Design review of the part built by this model. Coordinates are the model's own, in mm. Face numbers are marked on the shaded views. A direction names the side the tool comes from. Give positions to 0.01 mm unless a question says otherwise; leave off trailing zeros. Loops run counter-clockwise (first coordinate to the right, second up) from the corner with the lowest first, then second, coordinate; pieces in that order, holes last. Notation, with made-up numbers: (2.5, -38) - (53.5, -38) arc R6 cw to (53.5, -29) - close; hole circle Ø9 at (-9.5, -21.5). An arc over 180 degrees is marked (long way). Write each question's results on one line, items separated by ' | '.
```python
from build123d import *

# Parameters (mm, degrees)
SKETCH1_R               = 37.846
SKETCH1_R_2             = 14.224
BOSS_EXTRUDE1_DEPTH     = 6.35
CUT_EXTRUDE1_DEPTH      = 1
CUT_EXTRUDE1_DEPTH_BACK = 7.35
CUT_EXTRUDE2_DEPTH      = 1
CUT_EXTRUDE2_DEPTH_BACK = 7.35


with BuildPart() as part:
    # Sketch1 → Boss-Extrude1 (new body)
    with BuildSketch(Plane(origin=(0, 0, 0), x_dir=(1, 0, 0), z_dir=(0, 1, 0))):
        Circle(SKETCH1_R)
        Circle(SKETCH1_R_2, mode=Mode.SUBTRACT)
    extrude(amount=BOSS_EXTRUDE1_DEPTH)

    # Sketch2 → Cut-Extrude1 (cut, two sides)
    with BuildSketch(Plane(origin=(0, 6.35, 0), x_dir=(1, 0, 0), z_dir=(0, 1, 0))) as cut_extrude1_sk:
        Polygon((-18.723278008, -3.767243493), (-19.849678423, -4.7625), (-22.882156733, -4.7625), (-24.01035364, -3.767243493), (-24.01035364, -2.234835911), (-22.294703885, -2.234835911), (-22.294703885, -3.00373444), (-20.480247077, -3.00373444), (-20.480247077, -0.882077518), (-22.93605149, -0.882077518), (-24.058858921, 0.113178989), (-24.058858921, 3.761854017), (-22.93605149, 4.7625), (-19.862253866, 4.7625), (-18.723278008, 3.756464542), align=None)
        Polygon((-24.955308374, -3.767243493), (-26.083505281, -4.7625), (-29.139337986, -4.7625), (-30.267534892, -3.767243493), (-30.267534892, 3.761854017), (-29.151913429, 4.7625), (-26.1014702, 4.7625), (-24.973273293, 3.761854017), (-24.973273293, 2.288730668), (-26.737428329, 2.288730668), (-26.737428329, 3.00373444), (-28.508769332, 3.00373444), (-28.508769332, 0.882077518), (-26.083505281, 0.882077518), (-24.955308374, -0.105993022), align=None)
        Polygon((-31.110089589, -4.7625), (-32.868855149, -4.7625), (-32.868855149, 2.597727273), (-33.371872878, 2.597727273), (-33.371872878, 4.356492833), (-32.286791777, 4.7625), (-31.110089589, 4.7625), align=None)
        Polygon((20.831103766, 3.175), (22.005192308, 3.175), (22.005192308, -3.175), (21.435320513, -3.175), (21.435320513, 2.523717949), (20.458397436, 2.523717949), align=None)
        Polygon((27.703910256, 3.337820513), (25.047900641, -4.070512821), (24.4475, -4.070512821), (27.103509615, 3.337820513), align=None)
        Polygon((31.658667869, 3.337820513), (31.774423077, 3.337820513), (31.774423077, -1.058333333), (32.507115385, -1.058333333), (32.507115385, -1.709615385), (31.774423077, -1.709615385), (31.774423077, -3.175), (31.204551282, -3.175), (31.204551282, -1.709615385), (28.192371795, -1.709615385), align=None)
    extrude(amount=CUT_EXTRUDE1_DEPTH, mode=Mode.SUBTRACT)
    extrude(cut_extrude1_sk.sketch, amount=-CUT_EXTRUDE1_DEPTH_BACK, mode=Mode.SUBTRACT)

    # Sketch3 → Cut-Extrude2 (cut, two sides)
    with BuildSketch(Plane(origin=(0, 6.35, 0), x_dir=(1, 0, 0), z_dir=(0, 1, 0))) as cut_extrude2_sk:
        with BuildLine():
            Line((14.605, -10.631905207), (14.578021506, -10.616329166))
            ThreePointArc((14.578021506, -10.616329166), (9.017, -15.617902132), (1.905, -17.933101544))
            Line((1.905, -17.933101544), (1.905, -17.964253626))
            Line((1.905, -17.964253626), (8.255, -21.630427835))
            Line((8.255, -21.630427835), (14.605, -17.964253626))
            Line((14.605, -17.964253626), (14.605, -10.631905207))
        make_face()
        with BuildLine():
            ThreePointArc((-1.905, -17.933101544), (-9.017, -15.617902132), (-14.578021506, -10.616329166))
            Line((-14.578021506, -10.616329166), (-14.605, -10.631905207))
            Line((-14.605, -10.631905207), (-14.605, -17.964253626))
            Line((-14.605, -17.964253626), (-8.255, -21.630427835))
            Line((-8.255, -21.630427835), (-1.905, -17.964253626))
            Line((-1.905, -17.964253626), (-1.905, -17.933101544))
        make_face()
        with BuildLine():
            Line((29.197783942, -9.525), (20.332216058, -9.525))
            Line((20.332216058, -9.525), (18.415, -10.631905207))
            Line((18.415, -10.631905207), (18.415, -17.964253626))
            Line((18.415, -17.964253626), (24.765, -21.630427835))
            Line((24.765, -21.630427835), (27.504447445, -20.048807115))
            ThreePointArc((27.504447445, -20.048807115), (29.476040643, -17.018), (31.115, -13.795146647))
            Line((31.115, -13.795146647), (31.115, -10.631905207))
            Line((31.115, -10.631905207), (29.197783942, -9.525))
        make_face()
        with BuildLine():
            Line((-18.415, -10.631905207), (-20.332216058, -9.525))
            Line((-20.332216058, -9.525), (-29.197783942, -9.525))
            Line((-29.197783942, -9.525), (-31.115, -10.631905207))
            Line((-31.115, -10.631905207), (-31.115, -13.795146647))
            ThreePointArc((-31.115, -13.795146647), (-29.476040643, -17.018), (-27.504447445, -20.048807115))
            Line((-27.504447445, -20.048807115), (-24.765, -21.630427835))
            Line((-24.765, -21.630427835), (-18.415, -17.964253626))
            Line((-18.415, -17.964253626), (-18.415, -10.631905207))
        make_face()
        with BuildLine():
            ThreePointArc((1.905, 17.933101544), (8.977045814, 15.640901651), (14.523553183, 10.690723032))
            Line((14.523553183, 10.690723032), (14.605, 10.737746374))
            Line((14.605, 10.737746374), (14.605, 18.070094793))
            Line((14.605, 18.070094793), (8.255, 21.736269002))
            Line((8.255, 21.736269002), (1.905, 18.070094793))
            Line((1.905, 18.070094793), (1.905, 17.933101544))
        make_face()
        with BuildLine():
            Line((-14.605, 10.737746374), (-14.523553183, 10.690723032))
            ThreePointArc((-14.523553183, 10.690723032), (-8.977045814, 15.640901651), (-1.905, 17.933101544))
            Line((-1.905, 17.933101544), (-1.905, 18.070094793))
            Line((-1.905, 18.070094793), (-8.255, 21.736269002))
            Line((-8.255, 21.736269002), (-14.605, 18.070094793))
            Line((-14.605, 18.070094793), (-14.605, 10.737746374))
        make_face()
        with BuildLine():
            Line((18.415, 10.737746374), (20.515538337, 9.525))
            Line((20.515538337, 9.525), (29.014461663, 9.525))
            Line((29.014461663, 9.525), (31.115, 10.737746374))
            Line((31.115, 10.737746374), (31.115, 13.795146647))
            ThreePointArc((31.115, 13.795146647), (29.418907432, 17.11657622), (27.369604296, 20.232500011))
            Line((27.369604296, 20.232500011), (24.765, 21.736269002))
            Line((24.765, 21.736269002), (18.415, 18.070094793))
            Line((18.415, 18.070094793), (18.415, 10.737746374))
        make_face()
        with BuildLine():
            Line((-29.014461663, 9.525), (-20.515538337, 9.525))
            Line((-20.515538337, 9.525), (-18.415, 10.737746374))
            Line((-18.415, 10.737746374), (-18.415, 18.070094793))
            Line((-18.415, 18.070094793), (-24.765, 21.736269002))
            Line((-24.765, 21.736269002), (-27.369604296, 20.232500011))
            ThreePointArc((-27.369604296, 20.232500011), (-29.418907432, 17.11657622), (-31.115, 13.795146647))
            Line((-31.115, 13.795146647), (-31.115, 10.737746374))
            Line((-31.115, 10.737746374), (-29.014461663, 9.525))
        make_face()
        with BuildLine():
            ThreePointArc((10.290035143, -32.443250034), (16.964310844, -29.506972965), (22.86, -25.216456849))
            Line((22.86, -25.216456849), (22.86, -25.035825791))
            Line((22.86, -25.035825791), (16.51, -21.369651581))
            Line((16.51, -21.369651581), (10.16, -25.035825791))
            Line((10.16, -25.035825791), (10.16, -32.368174209))
            Line((10.16, -32.368174209), (10.290035143, -32.443250034))
        make_face()
        with BuildLine():
            Line((-22.86, -25.035825791), (-22.86, -25.216456849))
            ThreePointArc((-22.86, -25.216456849), (-16.964310844, -29.506972965), (-10.290035143, -32.443250034))
            Line((-10.290035143, -32.443250034), (-10.16, -32.368174209))
            Line((-10.16, -32.368174209), (-10.16, -25.035825791))
            Line((-10.16, -25.035825791), (-16.51, -21.369651581))
            Line((-16.51, -21.369651581), (-22.86, -25.035825791))
        make_face()
        with BuildLine():
            ThreePointArc((-3.837056844, -33.819022617), (0, -34.036), (3.837056844, -33.819022617))
            Line((3.837056844, -33.819022617), (6.35, -32.368174209))
            Line((6.35, -32.368174209), (6.35, -25.035825791))
            Line((6.35, -25.035825791), (0, -21.369651581))
            Line((0, -21.369651581), (-6.35, -25.035825791))
            Line((-6.35, -25.035825791), (-6.35, -32.368174209))
            Line((-6.35, -32.368174209), (-3.837056844, -33.819022617))
        make_face()
        with BuildLine():
            Line((22.86, 25.035825791), (22.86, 25.216456849))
            ThreePointArc((22.86, 25.216456849), (16.964310844, 29.506972965), (10.290035143, 32.443250034))
            Line((10.290035143, 32.443250034), (10.16, 32.368174209))
            Line((10.16, 32.368174209), (10.16, 25.035825791))
            Line((10.16, 25.035825791), (16.51, 21.369651581))
            Line((16.51, 21.369651581), (22.86, 25.035825791))
        make_face()
        with BuildLine():
            ThreePointArc((-10.290035143, 32.443250034), (-16.964310844, 29.506972965), (-22.86, 25.216456849))
            Line((-22.86, 25.216456849), (-22.86, 25.035825791))
            Line((-22.86, 25.035825791), (-16.51, 21.369651581))
            Line((-16.51, 21.369651581), (-10.16, 25.035825791))
            Line((-10.16, 25.035825791), (-10.16, 32.368174209))
            Line((-10.16, 32.368174209), (-10.290035143, 32.443250034))
        make_face()
        with BuildLine():
            Line((6.35, 32.368174209), (3.837056844, 33.819022617))
            ThreePointArc((3.837056844, 33.819022617), (0, 34.036), (-3.837056844, 33.819022617))
            Line((-3.837056844, 33.819022617), (-6.35, 32.368174209))
            Line((-6.35, 32.368174209), (-6.35, 25.035825791))
            Line((-6.35, 25.035825791), (0, 21.369651581))
            Line((0, 21.369651581), (6.35, 25.035825791))
            Line((6.35, 25.035825791), (6.35, 32.368174209))
        make_face()
    extrude(amount=CUT_EXTRUDE2_DEPTH, mode=Mode.SUBTRACT)
    extrude(cut_extrude2_sk.sketch, amount=-CUT_EXTRUDE2_DEPTH_BACK, mode=Mode.SUBTRACT)


solid = part.part
```
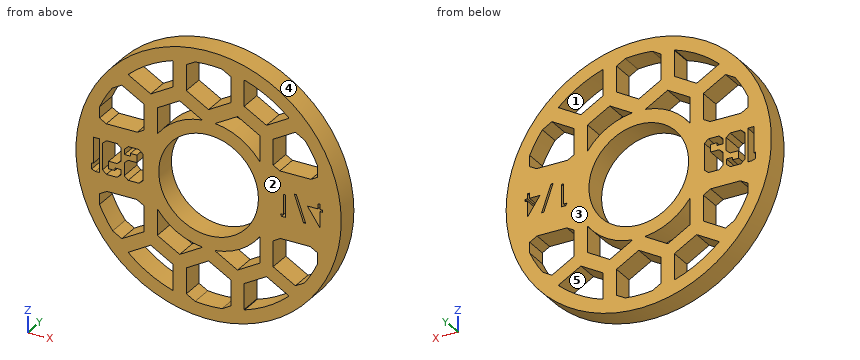
Item 1: We need section A-A on z = 30.5. Give the boundary of the cut face in (x, y), then the cut area to 3 significant figures.
Output values:
outline: (-22.41, 0) - (-15.11, 0) - (-15.11, 6.35) - (-22.41, 6.35) - close; (-10.16, 0) - (-6.35, 0) - (-6.35, 6.35) - (-10.16, 6.35) - close; (6.35, 0) - (10.16, 0) - (10.16, 6.35) - (6.35, 6.35) - close; (15.11, 0) - (22.41, 0) - (22.41, 6.35) - (15.11, 6.35) - close | area: 141 mm²
Item 2: Draft analysis for pull direction X (two halves, no side actions). For the marked faces 3, 4 and 5, state which applies: +X half, -X half, draft (parallel to the pull), parting line (faces both ways), or undercut.
Output values:
face 3: draft | face 4: parting line | face 5: undercut
Item 3: Tool access review of the marked faces 1 and 2: name each direction out of +Z, -Z, +X, -X, +Y, -Y from which nothing blocks a thin tool from reaching the whole face with its end or side.
Output values:
face 1: +Y, -Y | face 2: +Z, -Z, +X, -X, -Y
Item 4: We need section C-C on z = 6. Give the boundary of the cut face in (x, y), then the cut area to 3 significant figures.
Output values:
outline: (-37.37, 0) - (-12.9, 0) - (-12.9, 6.35) - (-37.37, 6.35) - close; (12.9, 0) - (37.37, 0) - (37.37, 6.35) - (12.9, 6.35) - close | area: 311 mm²
Item 5: Clearance check with flat-ended pins moving along their axes: P1, Ø1.9, axis at y = 3, z = 27.5, coming from the +X side; P2, Ø1, axis at x = -28.5, y = 3, coming from the +Z side; P3, Ø1.6, axis at y = 4.5, z = 2, coming from the -X side. State where each tip first meets the part, or that it passes through.
Output values:
P1: stops at x = 26.97 | P2: stops at z = 25.46 | P3: stops at x = -37.83
Item 6: We need section B-B on y = 1.5. Give the number of separate pieces and of enclosed holes in the cut face, then the cut area to 3 significant figures.
Output values:
separate pieces: 1 | enclosed holes: 21 | area: 2,450 mm²
Item 7: We need section D-D on z = -27.5. Give the boundary of the cut face in (x, y), then the cut area to 3 significant figures.
Output values:
outline: (-26, 0) - (-20.05, 0) - (-20.05, 6.35) - (-26, 6.35) - close; (-10.16, 0) - (-6.35, 0) - (-6.35, 6.35) - (-10.16, 6.35) - close; (6.35, 0) - (10.16, 0) - (10.16, 6.35) - (6.35, 6.35) - close; (20.05, 0) - (26, 0) - (26, 6.35) - (20.05, 6.35) - close | area: 124 mm²
Item 8: Wall thickness on probe 1 along Z at (x, y) = (0, 3.75); probe 2 along Z at (x, y) = (-15.5, 1.5); probe 3 along X at (y, z) = (5, 26): over which ranges is each line inside the solid? List them lowest first.
Output values:
probe 1: z = -37.85 to -34.04, -21.37 to -14.22, 14.22 to 21.37, 34.04 to 37.85 | probe 2: z = -34.53 to -30.3, -21.95 to 21.95, 30.3 to 34.53 | probe 3: x = -27.5 to -21.96, -10.16 to -6.35, 6.35 to 10.16, 21.96 to 27.5
